CAD build for the part. Positions are in the model's coordinates, mm. A direction names the side the tool comes from. Round coordinates to 2 decimals unless told otherwise and drop trailing zeros. Loops run counter-clockwise (first coordinate to the right, second up) from the corner with the lowest first, then second, coordinate; pieces in that order, holes last.
from build123d import *

# Parameters (mm, degrees)
BRIDA_BASE2_DEPTH       = 20
CORTAR_EXTRUIR1_START   = -20
CORTAR_EXTRUIR1_DEPTH   = 8
CORTAR_EXTRUIR1_START_2 = 17
CORTAR_EXTRUIR1_2_DEPTH = 3
CORTAR_EXTRUIR1_3_DEPTH = 3
CORTAR_EXTRUIR2_REACH   = 33.149
CROQUIS13_R             = 4.5
REDONDEO1_R             = 2


# Read off the part's stored shape, not the designer's step: Cortar-Extruir1
# Sheet-metal steps are written as plain solids
with BuildPart() as part:
    # Croquis9 → Brida base2 (new, symmetric)
    with BuildSketch(Plane.XY):
        with BuildLine():
            Line((-22.5, 0), (-11.295902805, 0))
            ThreePointArc((-11.295902805, 0), (-9.677249795, -0.368790327), (-8.378108412, -1.402364485))
            Line((-8.378108412, -1.402364485), (-5.721159702, -4.723550372))
            ThreePointArc((-5.721159702, -4.723550372), (-5.465058556, -4.927299964), (-5.145971737, -5))
            Line((-5.145971737, -5), (5.145971737, -5))
            ThreePointArc((5.145971737, -5), (5.465058556, -4.927299964), (5.721159702, -4.723550372))
            Line((5.721159702, -4.723550372), (8.378108412, -1.402364485))
            ThreePointArc((8.378108412, -1.402364485), (9.677249795, -0.368790327), (11.295902805, 0))
            Line((11.295902805, 0), (22.5, 0))
            Line((22.5, 0), (22.5, -3))
            Line((22.5, -3), (11.295902805, -3))
            ThreePointArc((11.295902805, -3), (10.976815986, -3.072700036), (10.72071484, -3.276449628))
            Line((10.72071484, -3.276449628), (8.063766131, -6.597635515))
            ThreePointArc((8.063766131, -6.597635515), (6.764624748, -7.631209673), (5.145971737, -8))
            Line((5.145971737, -8), (-5.145971737, -8))
            ThreePointArc((-5.145971737, -8), (-6.764624748, -7.631209673), (-8.063766131, -6.597635515))
            Line((-8.063766131, -6.597635515), (-10.72071484, -3.276449628))
            ThreePointArc((-10.72071484, -3.276449628), (-10.976815986, -3.072700036), (-11.295902805, -3))
            Line((-11.295902805, -3), (-22.5, -3))
            Line((-22.5, -3), (-22.5, 0))
        make_face()
    extrude(amount=BRIDA_BASE2_DEPTH, both=True)

    # Cortar-Extruir1 outline → Cortar-Extruir1 (cut)
    with BuildSketch(Plane.XY.offset(CORTAR_EXTRUIR1_START)):
        with BuildLine():
            Line((8.063766131, -6.597635515), (9.342606428, -4.999085143))
            Line((9.342606428, -4.999085143), (7, -3.125))
            Line((7, -3.125), (5.721159702, -4.723550372))
            ThreePointArc((5.721159702, -4.723550372), (5.465058556, -4.927299964), (5.145971737, -5))
            Line((5.145971737, -5), (-5.145971737, -5))
            ThreePointArc((-5.145971737, -5), (-5.465058556, -4.927299964), (-5.721159702, -4.723550372))
            Line((-5.721159702, -4.723550372), (-7, -3.125))
            Line((-7, -3.125), (-9.342606428, -4.999085143))
            Line((-9.342606428, -4.999085143), (-8.063766131, -6.597635515))
            ThreePointArc((-8.063766131, -6.597635515), (-6.764624748, -7.631209673), (-5.145971737, -8))
            Line((-5.145971737, -8), (5.145971737, -8))
            ThreePointArc((5.145971737, -8), (6.764624748, -7.631209673), (8.063766131, -6.597635515))
        make_face()
    extrude(amount=CORTAR_EXTRUIR1_DEPTH, mode=Mode.SUBTRACT)

    # Cortar-Extruir1 2 outline → Cortar-Extruir1 2 (cut)
    with BuildSketch(Plane.XY.offset(CORTAR_EXTRUIR1_START_2)):
        with BuildLine():
            Line((8.063766131, -6.597635515), (10.72071484, -3.276449628))
            ThreePointArc((10.72071484, -3.276449628), (10.82209851, -3.172606162), (10.941874542, -3.090656079))
            Line((10.941874542, -3.090656079), (9.5, -0.459877144))
            ThreePointArc((9.5, -0.459877144), (8.892404123, -0.8755908), (8.378108412, -1.402364485))
            Line((8.378108412, -1.402364485), (5.721159702, -4.723550372))
            ThreePointArc((5.721159702, -4.723550372), (5.465058556, -4.927299964), (5.145971737, -5))
            Line((5.145971737, -5), (-5.145971737, -5))
            ThreePointArc((-5.145971737, -5), (-5.465058556, -4.927299964), (-5.721159702, -4.723550372))
            Line((-5.721159702, -4.723550372), (-8.378108412, -1.402364485))
            ThreePointArc((-8.378108412, -1.402364485), (-8.892404123, -0.8755908), (-9.5, -0.459877144))
            Line((-9.5, -0.459877144), (-10.941874542, -3.090656079))
            ThreePointArc((-10.941874542, -3.090656079), (-10.82209851, -3.172606162), (-10.72071484, -3.276449628))
            Line((-10.72071484, -3.276449628), (-8.063766131, -6.597635515))
            ThreePointArc((-8.063766131, -6.597635515), (-6.764624748, -7.631209673), (-5.145971737, -8))
            Line((-5.145971737, -8), (5.145971737, -8))
            ThreePointArc((5.145971737, -8), (6.764624748, -7.631209673), (8.063766131, -6.597635515))
        make_face()
    extrude(amount=CORTAR_EXTRUIR1_2_DEPTH, mode=Mode.SUBTRACT)

    # Cortar-Extruir1 3 outline → Cortar-Extruir1 3 (cut)
    with BuildSketch(Plane.XY.offset(CORTAR_EXTRUIR1_START)):
        with BuildLine():
            Line((7, -3.125), (9.342606428, -4.999085143))
            Line((9.342606428, -4.999085143), (10.72071484, -3.276449628))
            ThreePointArc((10.72071484, -3.276449628), (10.82209851, -3.172606162), (10.941874542, -3.090656079))
            Line((10.941874542, -3.090656079), (9.5, -0.459877144))
            ThreePointArc((9.5, -0.459877144), (8.892404123, -0.8755908), (8.378108412, -1.402364485))
            Line((8.378108412, -1.402364485), (7, -3.125))
        make_face()
        with BuildLine():
            Line((-10.72071484, -3.276449628), (-9.342606428, -4.999085143))
            Line((-9.342606428, -4.999085143), (-7, -3.125))
            Line((-7, -3.125), (-8.378108412, -1.402364485))
            ThreePointArc((-8.378108412, -1.402364485), (-8.892404123, -0.8755908), (-9.5, -0.459877144))
            Line((-9.5, -0.459877144), (-10.941874542, -3.090656079))
            ThreePointArc((-10.941874542, -3.090656079), (-10.82209851, -3.172606162), (-10.72071484, -3.276449628))
        make_face()
    extrude(amount=CORTAR_EXTRUIR1_3_DEPTH, mode=Mode.SUBTRACT)

    # Croquis13 → Cortar-Extruir2 (cut, up to next)
    with BuildSketch(Plane(origin=(0, 0, 0), x_dir=(1, 0, 0), z_dir=(0, 1, 0)), mode=Mode.PRIVATE) as cortar_extruir2_sk1:
        with Locations(Location((-16, 12.5, 0), (0, 0, 270))):
            Circle(CROQUIS13_R)
    cortar_extruir2_tool1 = extrude(cortar_extruir2_sk1.sketch, amount=-CORTAR_EXTRUIR2_REACH, mode=Mode.PRIVATE) & part.part
    # Croquis13 → Cortar-Extruir2 (cut, up to next)
    with BuildSketch(Plane(origin=(0, 0, 0), x_dir=(1, 0, 0), z_dir=(0, 1, 0)), mode=Mode.PRIVATE) as cortar_extruir2_sk2:
        with Locations(Location((16, 12.5, 0), (0, 0, 270))):
            Circle(CROQUIS13_R)
    cortar_extruir2_tool2 = extrude(cortar_extruir2_sk2.sketch, amount=-CORTAR_EXTRUIR2_REACH, mode=Mode.PRIVATE) & part.part
    # Croquis13 → Cortar-Extruir2 (cut, up to next)
    with BuildSketch(Plane(origin=(0, 0, 0), x_dir=(1, 0, 0), z_dir=(0, 1, 0)), mode=Mode.PRIVATE) as cortar_extruir2_sk3:
        with Locations(Location((16, -12.5, 0), (0, 0, 270))):
            Circle(CROQUIS13_R)
    cortar_extruir2_tool3 = extrude(cortar_extruir2_sk3.sketch, amount=-CORTAR_EXTRUIR2_REACH, mode=Mode.PRIVATE) & part.part
    # Croquis13 → Cortar-Extruir2 (cut, up to next)
    with BuildSketch(Plane(origin=(0, 0, 0), x_dir=(1, 0, 0), z_dir=(0, 1, 0)), mode=Mode.PRIVATE) as cortar_extruir2_sk4:
        with Locations(Location((-16, -12.5, 0), (0, 0, 270))):
            Circle(CROQUIS13_R)
    cortar_extruir2_tool4 = extrude(cortar_extruir2_sk4.sketch, amount=-CORTAR_EXTRUIR2_REACH, mode=Mode.PRIVATE) & part.part
    add(cortar_extruir2_tool1.solids().sort_by_distance((-16, 0, -12.5))[0], mode=Mode.SUBTRACT)
    add(cortar_extruir2_tool2.solids().sort_by_distance((16, 0, -12.5))[0], mode=Mode.SUBTRACT)
    add(cortar_extruir2_tool3.solids().sort_by_distance((16, 0, 12.5))[0], mode=Mode.SUBTRACT)
    add(cortar_extruir2_tool4.solids().sort_by_distance((-16, 0, 12.5))[0], mode=Mode.SUBTRACT)

    # Redondeo1
    redondeo1_edges = [part.edges().sort_by_distance(p)[0] for p in [
        (22.5, -1.5, -20),
        (-22.5, -1.5, -20),
        (22.5, -1.5, 20),
        (-22.5, -1.5, 20),
    ]]
    fillet(redondeo1_edges, radius=REDONDEO1_R)


solid = part.part
Item 1: 3-axis set-ups, long thin cutter, end or side, ignore diameter. For faces 1 (the cylindrical face through (9.656, -0.379, 0.28)), 2 (the flat face through (10.23, -1.79, 18.48)), 3 (the flat face through (-10.211, -1.757, -18.521)): which of +Z, -Z, +X, -X, +Y, -Y reach the whole face in a straight line?
Verdict:
face 1: +Z, -Z, +Y
face 2: +Z, -Y
face 3: -Z, -Y
Item 2: Flat gauge pins, fed straight in: P1, Ø5, axis at x = 0, z = 6, coming from the +Y side; P2, Ø2, axis at x = 8.5, y = -2.5, coming from the -Z side; P3, Ø3, axis at y = -3.5, z = -7, coming from the +X side; P4, Ø12.5, axis at x = -16, z = 0, coming from the -Y side. Where does each tip first touch, or does it go through?
Verdict:
P1: stops at y = -5
P2: stops at z = -17
P3: stops at x = 22.5
P4: stops at y = -4.49
Item 3: Cut at C-C (z = 10). List the corners of the cut face in (x, y), plus the area to 3 significant figures.
Verdict:
outline: (-22.5, -3) - (-19.74, -3) - (-19.74, 0) - (-22.5, 0) - close; (-12.26, -3) - (-11.3, -3) arc R0.74 cw to (-10.72, -3.28) - (-8.06, -6.6) arc R3.74 ccw to (-5.15, -8) - (5.15, -8) arc R3.74 ccw to (8.06, -6.6) - (10.72, -3.28) arc R0.74 cw to (11.3, -3) - (12.26, -3) - (12.26, 0) - (11.3, 0) arc R3.74 ccw to (8.38, -1.4) - (5.72, -4.72) arc R0.74 cw to (5.15, -5) - (-5.15, -5) arc R0.74 cw to (-5.72, -4.72) - (-8.38, -1.4) arc R3.74 ccw to (-11.3, 0) - (-12.26, 0) - close; (19.74, -3) - (22.5, -3) - (22.5, 0) - (19.74, 0) - close
area: 103 mm2
Item 4: Cut at A-A (z = -12.5). List the corners of the cut face in (x, y) (3 decimals).
Verdict:
outline: (-22.5, -3) - (-20.5, -3) - (-20.5, 0) - (-22.5, 0) - close; (-11.5, -3) - (-11.296, -3) arc R0.737 cw to (-10.721, -3.276) - (-9.343, -4.999) - (-7, -3.125) - (-8.378, -1.402) arc R3.737 ccw to (-11.296, 0) - (-11.5, 0) - close; (7, -3.125) - (9.343, -4.999) - (10.721, -3.276) arc R0.737 cw to (11.296, -3) - (11.5, -3) - (11.5, 0) - (11.296, 0) arc R3.737 ccw to (8.378, -1.402) - close; (20.5, -3) - (22.5, -3) - (22.5, 0) - (20.5, 0) - close
Item 5: Cut at D-D (x = 10). List the corners of the cut face in (y, z).
Verdict:
outline: (-4.18, -17) - (-1.37, -17) - (-1.37, -20) - (-0.23, -20) - (-0.23, 20) - (-1.37, 20) - (-1.37, 17) - (-4.18, 17) - close
Item 6: Wall check: L1, parallel to X at y = -1.5, z = -13; L2, parallel to X at y = -2.3, z = -12.5; L3, parallel to Z at x = -3, y = -6.75. Give the ranges that are in metal, low to high.
Verdict:
L1: x = -22.5 to -20.47, -11.53 to -8.3, 8.3 to 11.53, 20.47 to 22.5
L2: x = -22.5 to -20.5, -11.5 to -7.66, 7.66 to 11.5, 20.5 to 22.5
L3: z = -12 to 17
Item 7: Cut at B-B (x = 16). List the corners of the cut face in (y, z), plus the area to 3 significant figures.
Verdict:
outline: (-3, -20) - (0, -20) - (0, -17) - (-3, -17) - close; (-3, -8) - (0, -8) - (0, 8) - (-3, 8) - close; (-3, 17) - (0, 17) - (0, 20) - (-3, 20) - close
area: 66.0 mm2
Item 8: Mould opens along X. For faces 4 (the flat face through (22.5, -1, 0)), 5 (the flat face through (-15, -2, 20)), 6 (the cylindrical face through (19.794, -1.479, -10.081)), 7 (the cylindrical face through (-12.206, -1.479, -10.081)) say: released by +X, released by -X, zero draft, split by the parting line, or undercut.
Verdict:
face 4: released by +X
face 5: zero draft
face 6: undercut
face 7: undercut
